Geometry check sheet. Reference: the model listing, model coordinates, mm. A direction names the side the tool comes from. Coordinates: 2 decimals unless noted, no trailing zeros. Order: outer loops, then holes, each group sorted by start corner. A loop starts at its lowest first (then second) coordinate and runs counter-clockwise, first axis right, second up. Notation, with made-up numbers: (30, -27) - (43, -27) arc R13 cw to (43, -14) - close; hole circle Ø1 at (-15.75, 11). An arc over 180 degrees is marked (long way). Return JSON: item names as keys, results as strings. Group by question number.
Item 1: Scan lines: probe 1 along Y at (x, z) = (0, 16.05); probe 2 along Y at (x, z) = (1.5, 16); probe 3 along Z at (x, y) = (0.85, -0.1). Record each from-to range of solid material in increasing order.
Item 2: Gauge pin test, flat end, axial feed: pin 1 (0.8 mm diameter, centred on x = -2, y = -0.5, fed in from +Z). Record the tip position at first contact, or that the pin passes through.
Item 3: Section check C-C on z = 15.5. Enter the section's corners in (x, y).
Item 4: Draft check along Y on faces 1 (the cylindrical face through (2.385, 0.751, 8.381)), 2 (the flat face through (0, 0, 15)), 3 (the flat face through (-1.5, 0, 12)). Enter one of: pulls with the +Y half, pulls with the -Y half, needs draft (parallel to the pull), parting line crosses it, or undercut.
Item 5: Section check A-A on x = 0. Enter the section's corners in (y, z), then the cut area to 3 significant figures.
Item 6: Section check D-D on z = 7.5. Enter the section's corners in (x, y).
Item 7: Tool access check on faces 4 (the cylindrical face through (0, -1, 16)), 5 (the flat face through (0, 0, 0)), 6 (the flat face through (-2, 0, 7)). Record the directions out of +Z, -Z, +X, -X, +Y, -Y that give a thin tool (end or side, any length) a straight path to the whole face; none if there is none.
Item 8: Section check B-B on y = 0. Enter the section's corners in (x, z).
from build123d import *

# Parameters (mm, degrees)
SKETCH1_R           = 2.5
BOSS_EXTRUDE1_DEPTH = 17
SKETCH2_W           = 1
SKETCH2_H           = 5
CUT_EXTRUDE1_DEPTH  = 10
SKETCH3_R           = 1
CUT_EXTRUDE2_DEPTH  = 2


with BuildPart() as part:
    # Sketch1 → Boss-Extrude1 (new body)
    with BuildSketch(Plane.XY):
        Circle(SKETCH1_R)
    extrude(amount=BOSS_EXTRUDE1_DEPTH)

    # Sketch2 → Cut-Extrude1 (cut)
    with BuildSketch(Plane.XY.offset(17)):
        with Locations((-2, 0)):
            Rectangle(SKETCH2_W, SKETCH2_H)
    extrude(amount=-CUT_EXTRUDE1_DEPTH, mode=Mode.SUBTRACT)

    # Sketch3 → Cut-Extrude2 (cut)
    with BuildSketch(Plane.XY.offset(17)):
        Circle(SKETCH3_R)
    extrude(amount=-CUT_EXTRUDE2_DEPTH, mode=Mode.SUBTRACT)


solid = part.part
Computed:
{
 "1": {"probe 1": "y = -2.5 to -1, 1 to 2.5", "probe 2": "y = -2 to 2", "probe 3": "z = 0 to 15"},
 "2": {"pin 1": "stops at z = 7"},
 "3": {"outline": "(-1.5, -2) arc R2.5 ccw (long way) to (-1.5, 2) - close; hole circle Ø2 at (0, 0)"},
 "4": {"face 1": "parting line crosses it", "face 2": "undercut", "face 3": "needs draft"},
 "5": {"outline": "(-2.5, 0) - (2.5, 0) - (2.5, 17) - (1, 17) - (1, 15) - (-1, 15) - (-1, 17) - (-2.5, 17) - close", "area": "81.0 mm²"},
 "6": {"outline": "(-1.5, -2) arc R2.5 ccw (long way) to (-1.5, 2) - close"},
 "7": {"face 4": "+Z", "face 5": "-Z, +X, -X, +Y, -Y", "face 6": "+Z, -X, +Y, -Y"},
 "8": {"outline": "(-2.5, 0) - (2.5, 0) - (2.5, 17) - (1, 17) - (1, 15) - (-1, 15) - (-1, 17) - (-1.5, 17) - (-1.5, 7) - (-2.5, 7) - close"}
}
